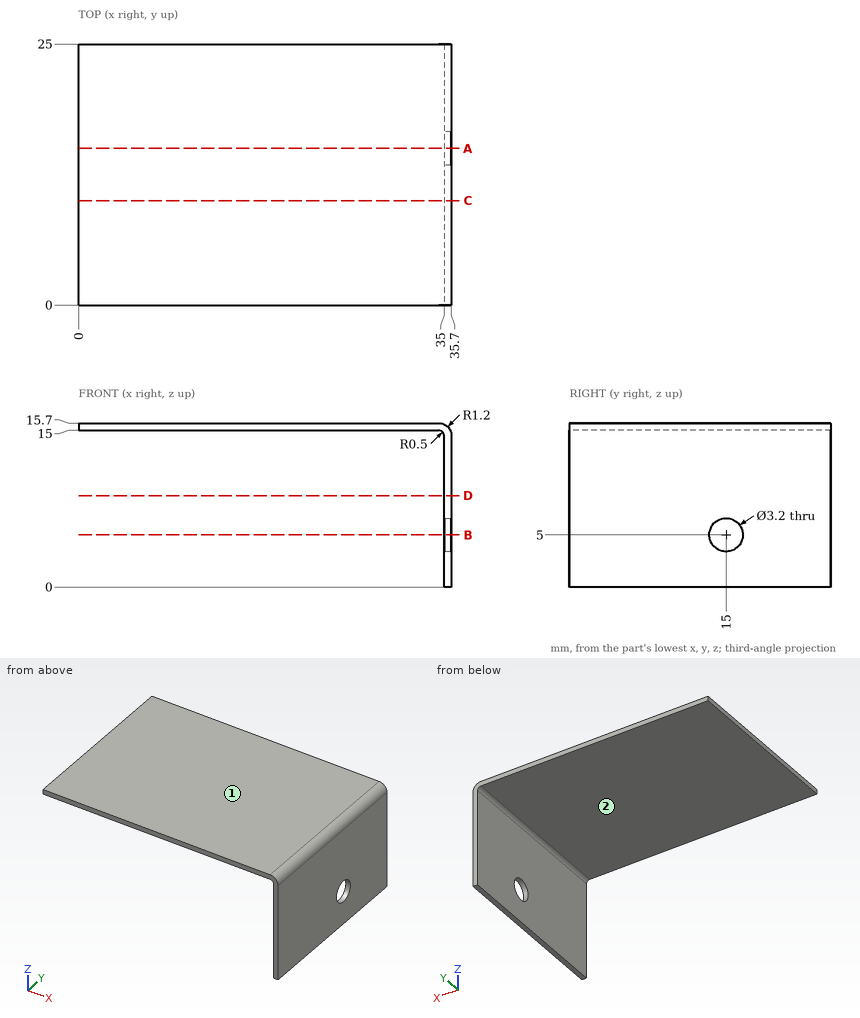
Study the drawing (mm; zero at the part's minimum x, y, z) and answer. A direction names the side the tool comes from. Round coordinates to 2 decimals unless told otherwise and drop trailing zeros. Loops run counter-clockwise (first coordinate to the right, second up) from the corner with the lowest first, then second, coordinate; pieces in that order, holes last.
Q1. Section D-D, the plane z = 8.75 is taken. Determine the outline of the cut face in (x, y).
Q2. Section B-B, the plane z = 5 is taken. Determine the outline of the cut face in (x, y), then the cut area to 3 significant figures.
Q3. Which of the six approach directions +Z, -Z, +X, -X, +Y, -Y give full straight-line access (tool end or side, diameter ignored) to the marked faces 1 and 2?
Q4. Find the intervals of material crossed by line 1 (Y direction, x = 35.5, z = 5); line 2 (X direction, y = 18, z = 7); line 3 (Z direction, x = 16, y = 13.75), in increasing order.
Q5. Section A-A, the plane y = 15 is taken. Determine the outline of the cut face in (x, z), then the cut area to 3 significant figures.
Q6. Section C-C, the plane y = 10 is taken. Determine the outline of the cut face in (x, z), then the cut area to 3 significant figures.
Q7. Given pin 1 Ø7 at (y, z) = (12, 5.5) entering from -X; pin 2 Ø12.5 at (x, y) = (9, 9.5) entering from -Z; pin 3 Ø4 at (y, z) = (15, 5) entering from +X, each flat-ended and moving along its own axis, determine where each tip first touches the part or whether it passes through.
Completed:
1. outline: (35, 0) - (35.7, 0) - (35.7, 25) - (35, 25) - close
2. outline: (35, 0) - (35.7, 0) - (35.7, 13.4) - (35, 13.4) - close; (35, 16.6) - (35.7, 16.6) - (35.7, 25) - (35, 25) - close
2. area: 15.3 mm2
3. face 1: +Z, +X, -X, +Y, -Y
3. face 2: -Z, -X, +Y, -Y
4. line 1: y = 0 to 13.4, 16.6 to 25
4. line 2: x = 35 to 35.7
4. line 3: z = 15 to 15.7
5. outline: (0, 15) - (34.5, 15) arc R0.5 cw to (35, 14.5) - (35, 6.6) - (35.7, 6.6) - (35.7, 14.5) arc R1.2 ccw to (34.5, 15.7) - (0, 15.7) - close; (35, 0) - (35.7, 0) - (35.7, 3.4) - (35, 3.4) - close
5. area: 33.0 mm2
6. outline: (0, 15) - (34.5, 15) arc R0.5 cw to (35, 14.5) - (35, 0) - (35.7, 0) - (35.7, 14.5) arc R1.2 ccw to (34.5, 15.7) - (0, 15.7) - close
6. area: 35.2 mm2
7. pin 1: stops at x = 35
7. pin 2: stops at z = 15
7. pin 3: stops at x = 35.7
